Geometry check sheet. Reference: the model listing, model coordinates, mm. A direction names the side the tool comes from. Round coordinates to 2 decimals unless told otherwise and drop trailing zeros. Loops run counter-clockwise (first coordinate to the right, second up) from the corner with the lowest first, then second, coordinate; pieces in that order, holes last. Notation, with made-up numbers: (-11, 47.5) - (-5, 47.5) arc R13 ccw to (-5, 60.5) - close; hole circle Ø8 at (39.5, -26). An arc over 180 degrees is marked (long way). Answer in a Markdown table with one row per item. Add a question column.
Autodesk Inventor part; units mm, degrees
ref_plane "YZ Plane" through (0, 0, 0) normal (1, 0, 0) x (0, 1, 0)
ref_plane "XZ Plane" through (0, 0, 0) normal (0, 1, 0) x (-1, 0, 0)
ref_plane "XY Plane" through (0, 0, 0) normal (0, 0, 1) x (1, 0, 0)
ref_plane "Work Plane1" through (0, 0, 0) normal (0, 0, 1) x (1, 0, 0)
sketch "Sketch1" plane through (0, 0, 0) normal (0, 0, 1) x (1, 0, 0)
  circle A0 centre (15, 28) radius 2.45
  circle A1 centre (-15, 28) radius 2.45
  circle A2 centre (0, -26.0002) radius 2.45
  line L0 (-22.5, -35) -> (22.5, -35)
  line L1 (22.5, -35) -> (22.5, 35)
  line L2 (22.5, 35) -> (-22.5, 35)
  line L3 (-22.5, 35) -> (-22.5, -35)
  line L4 (-22.5, -35) -> (22.5, 35) construction
  line L5 (22.5, -35) -> (-22.5, 35) construction
  line L6 (-15, -7.5) -> (15, -7.5)
  line L7 (15, -7.5) -> (15, 7.5)
  line L8 (15, 7.5) -> (-15, 7.5)
  line L9 (-15, 7.5) -> (-15, -7.5)
  line L10 (-15, -7.5) -> (15, 7.5) construction
  line L11 (15, -7.5) -> (-15, 7.5) construction
  point P0 (0, 0)
  dimension "d0" = 45
  dimension "d1" = 70
  dimension "d2" = 30
  dimension "d3" = 15
extrude "Extrusion1" add sketch "Sketch1" along normal blind 4
sketch "Sketch2" plane through (0, 0, 4) normal (0, 0, 1) x (1, 0, 0)
  point P0 (0, 0)
sketch "Sketch3" plane through (0, 0, 4) normal (0, 0, 1) x (1, 0, 0)
  line L0 (-15, -7.5) -> (-15, 7.5)
  line L1 (-15, 7.5) -> (15, 7.5)
  line L2 (15, 7.5) -> (15, -7.5)
  line L3 (15, -7.5) -> (-15, -7.5)
  circle A0 centre (0, -26.0002) radius 2.45
  circle A1 centre (-15, 28) radius 2.45
  circle A2 centre (15, 28) radius 2.45
  line L4 (-22.5, -35) -> (22.5, -35)
  line L5 (22.5, -35) -> (22.5, 35)
  line L6 (22.5, 35) -> (-22.5, 35)
  line L7 (-22.5, 35) -> (-22.5, -35)
  point P0 (0, 0)
extrude "Extrusion2" add sketch "Sketch3" along normal blind 1 contours A0 | A1 | A2 | L7 L6 L5 L4
sketch "Sketch4" plane through (0, 0, 5) normal (0, 0, 1) x (1, 0, 0)
  line L0 (-15, -9.25) -> (15, -9.25)
  line L1 (15, -9.25) -> (15, 9.25)
  line L2 (15, 9.25) -> (-15, 9.25)
  line L3 (-15, 9.25) -> (-15, -9.25)
  line L4 (-15, -9.25) -> (15, 9.25) construction
  line L5 (15, -9.25) -> (-15, 9.25) construction
  point P0 (0, 0)
  dimension "d8" = 30
  dimension "d9" = 18.5
extrude "Extrusion3" cut sketch "Sketch4" against normal blind 4.5
properties part number "03_MountCoverslip"
Q1. Cross-section at A-A, the plane y = -2. Enter the section's corners in (x, z), plus the area to 3 significant figures.
Q2. Scan lines: line 1 (Y direction, x = 0, z = 3.1); line 2 (Y direction, x = -6.5, z = 2.4); line 3 (X direction, y = -2.5, z = 2.85). Record each from-to range of solid material in increasing order. Write a range as from..to.
Q3. Release check for a two-part mould opening along X. For faces 4 (the flat face through (-22.5, 0, 2)), 5 (the flat face through (0, 8, 0)), 6 (the cylindrical face through (-16.806, 26.344, 1.972)) record: +X half, -X half, draft (parallel to the pull), parting line (faces both ways), or undercut.
Q4. Cross-section at B-B, the plane x = -8.5. Enter the section's corners in (y, z), plus the area to 3 significant figures.
Q5. Cross-section at C-C, the plane z = 1.5. Enter the section's corners in (x, y).
Q6. Depth check by flat-ended pin: P1, Ø2.5, axis at x = 0.5, y = -26, coming from the -Z side; P2, Ø6, axis at x = 0, y = 7, coming from the -Z side; P3, Ø0.5, axis at x = -3, y = -8, coming from the +Z side; P4, Ø1.5, axis at x = 13, y = -6, coming from the +Z side. Enter the tip coordinate at first touch or a pass-through.
Q7. Cross-section at D-D, the plane y = 28. Enter the section's corners in (x, z).
Q8. Set-up check for faces 1 (the flat face through (0, -35, 2)), 2 (the flat face through (15, 28, 4)), 3 (the flat face through (15, 0, 2)): record each of +Z, -Z, +X, -X, +Y, -Y from which the full face is reachable in a straight line by a thin tool's end or side.
Check sheet entries:
| question | item | result |
|---|---|---|
| 1 | outline | (-22.5, 0) - (-15, 0) - (-15, 5) - (-22.5, 5) - close; (15, 0) - (22.5, 0) - (22.5, 5) - (15, 5) - close |
| 1 | area | 75.0 mm² |
| 2 | line 1 | -35..-28.45, -23.55..-9.25, 9.25..35 |
| 2 | line 2 | -35..-9.25, 9.25..35 |
| 2 | line 3 | -22.5..-15, 15..22.5 |
| 3 | face 4 | -X half |
| 3 | face 5 | draft |
| 3 | face 6 | undercut |
| 4 | outline | (-35, 0) - (-7.5, 0) - (-7.5, 0.5) - (-9.25, 0.5) - (-9.25, 5) - (-35, 5) - close; (7.5, 0) - (35, 0) - (35, 5) - (9.25, 5) - (9.25, 0.5) - (7.5, 0.5) - close |
| 4 | area | 259 mm² |
| 5 | outline | (-22.5, -35) - (22.5, -35) - (22.5, 35) - (-22.5, 35) - close; hole circle Ø4.9 at (-15, 28); hole (-15, -9.25) - (15, -9.25) - (15, 9.25) - (-15, 9.25) - close; hole circle Ø4.9 at (0, -26); hole circle Ø4.9 at (15, 28) |
| 6 | P1 | z = 4 |
| 6 | P2 | z = 0 |
| 6 | P3 | z = 0.5 |
| 6 | P4 | through |
| 7 | outline | (-22.5, 0) - (-17.45, 0) - (-17.45, 4) - (-12.55, 4) - (-12.55, 0) - (12.55, 0) - (12.55, 4) - (17.45, 4) - (17.45, 0) - (22.5, 0) - (22.5, 5) - (-22.5, 5) - close |
| 8 | face 1 | +Z, -Z, +X, -X, -Y |
| 8 | face 2 | -Z |
| 8 | face 3 | +Z |
